Geometry: final body of the model. Coordinates: model frame, mm. Coordinates: 2 decimals unless noted, no trailing zeros. Loops run counter-clockwise (first coordinate to the right, second up) from the corner with the lowest first, then second, coordinate; pieces in that order, holes last. Notation, with made-up numbers: (-39, 35.5) - (-23, 35.5) arc R18 cw to (-23, 59.5) - close; hole circle Ø10 at (1, 6.25). An arc over 180 degrees is marked (long way). Answer in a Markdown table with one row per item.
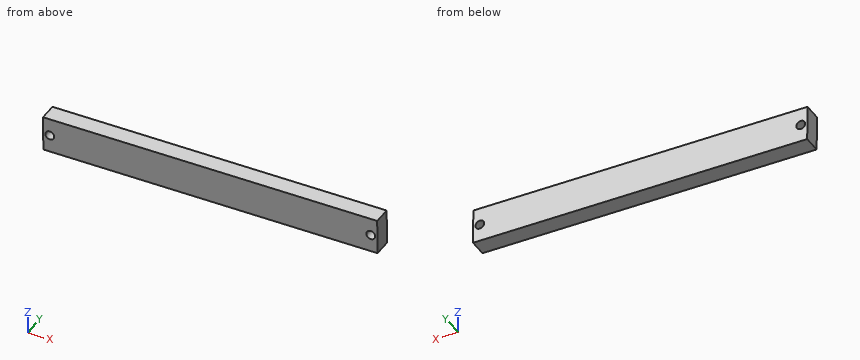
from build123d import *

# Parameters (mm, degrees)
F1_DEPTH = 12.7
F3_DEPTH = 12.701


with BuildPart() as f1:
    # F0 (on Front) → F1 (new body)
    with BuildSketch(Plane.XZ):
        Polygon((157.966793, 14.448158), (-83.321497, 12.070934), (-83.071263, -13.327833), (158.217027, -10.950609), align=None)
    extrude(amount=F1_DEPTH)

    # F2 (on face) → F3 (cut, through all)
    with BuildSketch(Plane.XZ.offset(12.7)):
        with BuildLine():
            ThreePointArc((-81.608957, -0.61281), (-78.418471, -3.756492), (-75.259111, -0.58153))
            ThreePointArc((-75.259111, -0.58153), (-78.449751, 2.593431), (-81.608957, -0.61281))
        make_face()
        with BuildLine():
            ThreePointArc((156.504487, 1.733135), (150.15468, 1.686216), (156.504641, 1.701856))
            ThreePointArc((156.504641, 1.701856), (156.504603, 1.717496), (156.504487, 1.733135))
        make_face()
    extrude(amount=-F3_DEPTH, mode=Mode.SUBTRACT)


solid = f1.part
(1) Cut plane A-A on y = -6. State how many separate pieces and enclosed holes the cut face has, then the cut area to 3 significant figures.
Verdict:
| item | result |
|---|---|
| separate pieces | 1 |
| enclosed holes | 2 |
| area | 6,070 mm² |
(2) Ray query, probe 1 along X at (y, z) = (-6, 0); probe 2 along X at (y, z) = (-0.75, 10.5); probe 3 along X at (y, z) = (-1.25, 4.5). Return the intervals inside material, ascending.
Verdict:
| item | result |
|---|---|
| probe 1 | x = -83.2 to -81.56, -75.31 to 150.65, 156.01 to 158.11 |
| probe 2 | x = -83.31 to 158.01 |
| probe 3 | x = -83.25 to 151.83, 154.83 to 158.06 |
(3) First-contact query: pin 1 Ø1.5 at (y, z) = (-8, 9.5) entering from -X; pin 2 Ø1 at (y, z) = (-2.5, -6.5) entering from -X; pin 3 Ø6 at (x, y) = (25, -3.5) entering from -Z. Flat tips, straight axial feed; report the tip coordinate or a pass-through.
Verdict:
| item | result |
|---|---|
| pin 1 | stops at x = -83.3 |
| pin 2 | stops at x = -83.14 |
| pin 3 | stops at z = -12.29 |
(4) Cut plane B-B on x = 108. Output: boundary loops of the cut face in (y, z).
Verdict:
| item | result |
|---|---|
| outline | (-12.7, -11.45) - (0, -11.45) - (0, 13.96) - (-12.7, 13.96) - close |
